Read the model definition and answer for the solid it produces. Units are mm, in the model's axes. Face numbers are marked on the shaded views. A direction names the side the tool comes from. Coordinates: 2 decimals unless noted, no trailing zeros. Write each loop counter-clockwise with the first axis right and the second up, starting at its lowest first coordinate (ties: lowest second). Pieces come first, ordered by that corner, then holes. Notation, with made-up numbers: (65.25, 52) -> (81.25, 52) arc R29 cw to (81.25, 76) -> close; hole circle Ø8 at (84, -18.5). An arc over 180 degrees is marked (long way). Use CSV: the item, a comma, the result in double quotes.
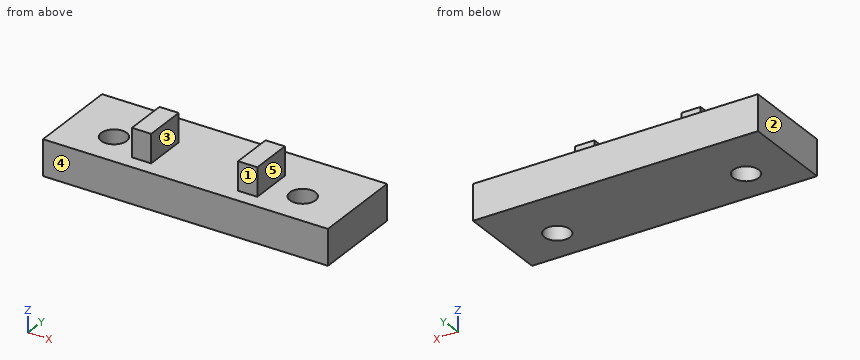
from build123d import *

# Parameters (mm, degrees)
SKETCH1_W            = 40
SKETCH1_H            = 10
BOSS_EXTRUDE1_DEPTH  = 5
M3_CLEARANCE_HOLE1_D = 3.6
SKETCH4_W            = 2.7
SKETCH4_H            = 6
BOSS_EXTRUDE2_DEPTH  = 4
SKETCH5_W            = 40
SKETCH5_H            = 5
BOSS_EXTRUDE3_DEPTH  = 2.9


with BuildPart() as part:
    # Sketch1 → Boss-Extrude1 (new body)
    with BuildSketch(Plane.XY):
        Rectangle(SKETCH1_W, SKETCH1_H)
    extrude(amount=BOSS_EXTRUDE1_DEPTH)

    # M3 Clearance Hole1 (through all)
    with Locations(Plane(origin=(0, 0, 0), x_dir=(1, 0, 0), z_dir=(0, 0, -1))):
        with Locations((-13.25, 0), (13.25, 0)):
            Hole(M3_CLEARANCE_HOLE1_D / 2)

    # Sketch4 → Boss-Extrude2 (add)
    with BuildSketch(Plane.XY.offset(5)):
        with Locations((-7.45, 0)):
            Rectangle(SKETCH4_W, SKETCH4_H)
        with Locations((7.45, 0)):
            Rectangle(SKETCH4_W, SKETCH4_H)
    extrude(amount=BOSS_EXTRUDE2_DEPTH)

    # Sketch5 → Boss-Extrude3 (add)
    with BuildSketch(Plane(origin=(0, 5, 0), x_dir=(1, 0, 0), z_dir=(0, 1, 0))):
        with Locations((0, -2.5)):
            Rectangle(SKETCH5_W, SKETCH5_H)
    extrude(amount=BOSS_EXTRUDE3_DEPTH)


solid = part.part
1. Find the intervals of material crossed by line 1 along Y through (x, z) = (13.25, 2.8); line 2 along X through (y, z) = (1, 4.25); line 3 along X through (y, z) = (2, 8.5), in increasing order.
Solutions:
line 1,"y = -5 to -1.8, 1.8 to 7.9"
line 2,"x = -20 to -14.75, -11.75 to 11.75, 14.75 to 20"
line 3,"x = -8.8 to -6.1, 6.1 to 8.8"
2. A cutting plane is placed at D-D (z = 1.5). Give the vertices of the cut face in (x, y).
Solutions:
outline,"(-20, -5) -> (20, -5) -> (20, 7.9) -> (-20, 7.9) -> close; hole circle Ø3.6 at (-13.25, 0); hole circle Ø3.6 at (13.25, 0)"
3. A cutting plane is placed at A-A (x = -13.25). Give the vertices of the cut face in (y, z), and give its area (3 significant figures).
Solutions:
outline,"(-5, 0) -> (-1.8, 0) -> (-1.8, 5) -> (-5, 5) -> close; (1.8, 0) -> (7.9, 0) -> (7.9, 5) -> (1.8, 5) -> close"
area,"46.5 mm^2"
4. A cutting plane is placed at C-C (z = 5.75). Give the vertices of the cut face in (x, y).
Solutions:
outline,"(-8.8, -3) -> (-6.1, -3) -> (-6.1, 3) -> (-8.8, 3) -> close; (6.1, -3) -> (8.8, -3) -> (8.8, 3) -> (6.1, 3) -> close"
5. For a pull along X with two mould halves and no side action, classify the marked faces 3, 4 and 5 as pulls with the +X half, pulls with the -X half, needs draft (parallel to the pull), parting line crosses it, or undercut.
Solutions:
face 3,"undercut"
face 4,"needs draft"
face 5,"pulls with the +X half"
6. A tool of negligible diameter and unlimited length cuts with its end or side. For the marked faces 1 and 2, from which of +Z, -Z, +X, -X, +Y, -Y can it reach the whole face along a straight path? Write none if from no direction.
Solutions:
face 1,"+Z, +X, -X, -Y"
face 2,"+Z, -Z, -X, +Y, -Y"
7. A cutting plane is placed at B-B (y = 0). Give the vertices of the cut face in (x, z), and give its area (3 significant figures).
Solutions:
outline,"(-20, 0) -> (-15.05, 0) -> (-15.05, 5) -> (-20, 5) -> close; (-11.45, 0) -> (11.45, 0) -> (11.45, 5) -> (8.8, 5) -> (8.8, 9) -> (6.1, 9) -> (6.1, 5) -> (-6.1, 5) -> (-6.1, 9) -> (-8.8, 9) -> (-8.8, 5) -> (-11.45, 5) -> close; (15.05, 0) -> (20, 0) -> (20, 5) -> (15.05, 5) -> close"
area,"186 mm^2"
8. Each of these flat-tipped pins is pushed along its axis until it touches: pin 1 Ø6 at (x, y) = (-3, -3) entering from +Z; pin 2 Ø3 at (x, z) = (8, 7) entering from -Y; pin 3 Ø1.4 at (x, z) = (7, 7) entering from +Y. Where does it stop, or does it pass through?
Solutions:
pin 1,"stops at z = 5"
pin 2,"stops at y = -3"
pin 3,"stops at y = 3"
